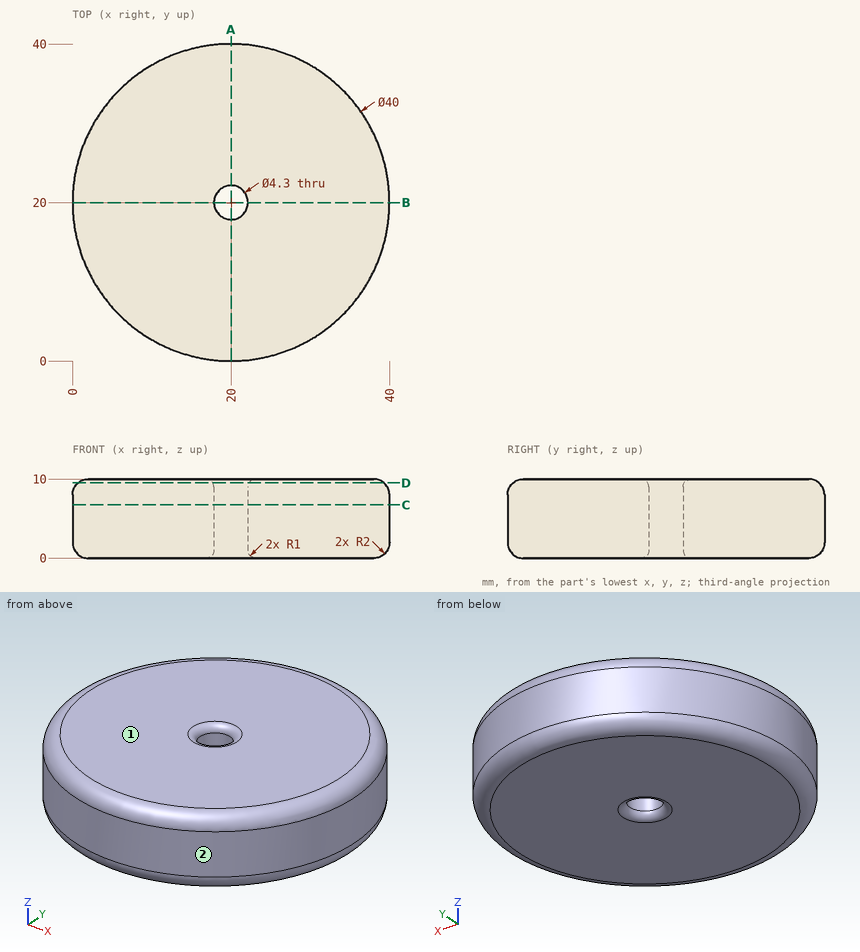
Print and shaded views of the part. All mm, measured from the part's lowest x, y and z. Round coordinates to 2 decimals unless told otherwise and drop trailing zeros. Write each loop counter-clockwise with the first axis right and the second up, starting at its lowest first coordinate (ties: lowest second). Pieces come first, ordered by that corner, then holes. Notation, with made-up numbers: (32, 84) - (59, 84) arc R13 cw to (59, 94) - close; hole circle Ø11 at (-23, -33). An arc over 180 degrees is marked (long way). One line per item, written item: value.
(1) Cut at A-A, the plane x = 20. Give the cut face in (y, z), plus the area to 3 significant figures.
Values follow:
outline: (0, 2) arc R2 ccw to (2, 0) - (16.85, 0) arc R1 ccw to (17.85, 1) - (17.85, 9) arc R1 ccw to (16.85, 10) - (2, 10) arc R2 ccw to (0, 8) - close; (22.15, 1) arc R1 ccw to (23.15, 0) - (38, 0) arc R2 ccw to (40, 2) - (40, 8) arc R2 ccw to (38, 10) - (23.15, 10) arc R1 ccw to (22.15, 9) - close
area: 353 mm²
(2) Cut at C-C, the plane z = 6.75. Give the cut face in (x, y), plus the area to 3 significant figures.
Values follow:
outline: circle Ø40 at (20, 20); hole circle Ø4.3 at (20, 20)
area: 1,240 mm²
(3) Wall check: probe 1 along Y at (x, z) = (20, 3.5); probe 2 along Z at (x, y) = (11.5, 36); probe 3 along X at (y, z) = (21, 1.5). Give the ranges that are in metal, low to high.
Values follow:
probe 1: y = 0 to 17.85, 22.15 to 40
probe 2: z = 0 to 10
probe 3: x = 0.09 to 18.1, 21.9 to 39.91
(4) Drop flat-ended pins along their axis: P1, Ø3, axis at y = 25, z = 8, coming from the -X side; P2, Ø7, axis at x = 20, y = 20, coming from the -Z side; P3, Ø2, axis at y = 22.5, z = 7.5, coming from the -X side; P4, Ø1, axis at x = 17.5, z = 5, coming from the -Y side. Give the stop position or say it passes through.
Values follow:
P1: stops at x = 0.31
P2: stops at z = 0
P3: stops at x = 0.06
P4: stops at y = 0.1
(5) Cut at D-D, the plane z = 9.5. Give the cut face in (x, y), plus the area to 3 significant figures.
Values follow:
outline: circle Ø38.65 at (20, 20); hole circle Ø4.57 at (20, 20)
area: 1,160 mm²
(6) Two-plate mould, pull along Y, no slides. Class the marked faces 1 and 2: pulls with the +Y half, pulls with the -Y half, needs draft (parallel to the pull), parting line crosses it, or undercut.
Values follow:
face 1: needs draft
face 2: parting line crosses it
